The model under review builds one solid part; all positions refer to its coordinate system, in mm. Round coordinates to 2 decimals unless told otherwise and drop trailing zeros. Loops run counter-clockwise (first coordinate to the right, second up) from the corner with the lowest first, then second, coordinate; pieces in that order, holes last. Notation, with made-up numbers: M 4,-33.5 L 27,-33.5 A37 ccw 27,3.5 Z; hole C 30,32 d5. An arc over 180 degrees is marked long. Answer in a Markdown table with one row per item. Add a question column.
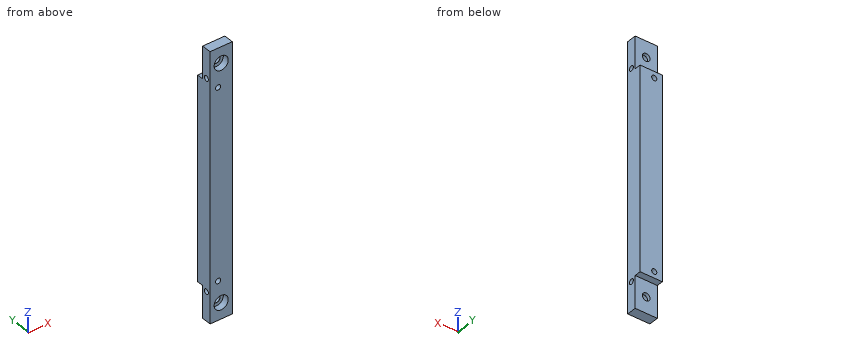
from build123d import *

# Parameters (mm, degrees)
SKETCH1_W                                      = 83
SKETCH1_H                                      = 6
BOSS_EXTRUDE1_DEPTH                            = 8.5
SKETCH7_W                                      = 8.5
SKETCH7_H                                      = 10
CUT_EXTRUDE6_DEPTH                             = 3
SKETCH18_W                                     = 10
SKETCH18_H                                     = 3
CUT_EXTRUDE8_DEPTH                             = 10
SKETCH21_W                                     = 63
SKETCH21_H                                     = 1
CUT_EXTRUDE9_DEPTH                             = 10
M2X0_4_TAPPED_HOLE3_D                          = 1.6
SKETCH27_W                                     = 1.6
SKETCH27_H                                     = 83
CUT_EXTRUDE12_DEPTH                            = 10
CBORE_FOR_M2_SOCKET_HEAD_CAP_SCREW1_AT_2_COUNT = 2
CBORE_FOR_M2_SOCKET_HEAD_CAP_SCREW1_AT_2_PITCH = 73
M2X0_4_TAPPED_HOLE2_D                          = 1.6


with BuildPart() as part:
    # Sketch1 → Boss-Extrude1 (new body)
    with BuildSketch(Plane(origin=(0, 0, 0), x_dir=(0, 0, -1), z_dir=(1, 0, 0))):
        with Locations((41.5, -5.098419508)):
            Rectangle(SKETCH1_W, SKETCH1_H)
    extrude(amount=BOSS_EXTRUDE1_DEPTH)

    # Sketch7 → Cut-Extrude6 (cut)
    with BuildSketch(Plane(origin=(0, -2.098419508, 0), x_dir=(1, 0, 0), z_dir=(0, 1, 0))):
        with Locations((4.25, 5)):
            Rectangle(SKETCH7_W, SKETCH7_H)
    extrude(amount=-CUT_EXTRUDE6_DEPTH, mode=Mode.SUBTRACT)

    # Sketch18 → Cut-Extrude8 (cut)
    with BuildSketch(Plane(origin=(8.5, 0, 0), x_dir=(0, 0, -1), z_dir=(1, 0, 0))):
        with Locations((78, -3.598419508)):
            Rectangle(SKETCH18_W, SKETCH18_H)
    extrude(amount=-CUT_EXTRUDE8_DEPTH, mode=Mode.SUBTRACT)

    # Sketch21 → Cut-Extrude9 (cut)
    with BuildSketch(Plane.ZY):
        with Locations((-41.5, -2.598419508)):
            Rectangle(SKETCH21_W, SKETCH21_H)
    extrude(amount=-CUT_EXTRUDE9_DEPTH, mode=Mode.SUBTRACT)

    # M2x0.4 Tapped Hole3 (through all)
    with Locations(Plane.ZY):
        with Locations((-74, -6.598419508), (-9, -6.598419508)):
            Hole(M2X0_4_TAPPED_HOLE3_D / 2)

    # Sketch27 → Cut-Extrude12 (cut)
    with BuildSketch(Plane.XZ.offset(8.098419508)):
        with Locations((0.8, -41.5)):
            Rectangle(SKETCH27_W, SKETCH27_H)
    extrude(amount=-CUT_EXTRUDE12_DEPTH, mode=Mode.SUBTRACT)

    # Sketch31 → CBORE for M2 Socket Head Cap Screw1 (revolve, cut)
    with BuildSketch(Plane(origin=(5.05, -8.098419508, -5), x_dir=(0, 0, -1), z_dir=(1, 0, 0))):
        Polygon((0, 0), (0, 5), (1.2, 5), (1.2, 2.025), (1.225, 2), (2.2, 2), (2.2, 0), align=None)
    cbore_for_m2_socket_head_cap_screw1 = revolve(axis=Axis((5.05, -14.448419508, -5), (0, 1, 0)), mode=Mode.SUBTRACT)

    # CBORE for M2 Socket Head Cap Screw1 at 2: CBORE for M2 Socket Head Cap Screw1 ×2
    with Locations(*[(0, 0, -i * CBORE_FOR_M2_SOCKET_HEAD_CAP_SCREW1_AT_2_PITCH) for i in range(1, CBORE_FOR_M2_SOCKET_HEAD_CAP_SCREW1_AT_2_COUNT)]):
        add(cbore_for_m2_socket_head_cap_screw1, mode=Mode.SUBTRACT)

    # M2x0.4 Tapped Hole2 (through all)
    with Locations(Plane(origin=(0, -8.098419508, 0), x_dir=(-1, 0, 0), z_dir=(0, -1, 0))):
        with Locations((-4.1, 71), (-4.1, 12)):
            Hole(M2X0_4_TAPPED_HOLE2_D / 2)


solid = part.part
1. Take a section at B-B, the plane y = -3.9. State the section outline as (x, z) points.
2. To check wall thickness, follow probe 1 along Z at (x, y) = (4.1, -5); probe 2 along Z at (x, y) = (5.05, -5.7); probe 3 along Z at (x, y) = (5.05, -6.5). State the ranges of each line that lie inside material, in increasing order.
3. Take a section at A-A, the plane z = -71. State the section outline as (x, y) points, and give its area (3 significant figures).
4. Take a section at C-C, the plane z = -5. State the section outline as (x, y) points (3 decimals).
5. For pin 1 Ø2 at (x, y) = (4, -4) entering from +Z; pin 2 Ø4 at (x, z) = (5.05, -5) entering from -Y; pin 3 Ø2 at (x, y) = (4, -4) entering from -Z, all flat-tipped, find the tip position at first contact; note any pin that passes through.
Check sheet entries:
| question | item | result |
|---|---|---|
| 1 | outline | M 1.6,-73 L 8.5,-73 L 8.5,-10 L 1.6,-10 Z; hole C 4.1,-71 d1.6; hole C 4.1,-12 d1.6 |
| 2 | probe 1 | z = -73 to -71.8, -70.2 to -12.8, -11.2 to -10 |
| 2 | probe 2 | z = -83 to -79.2, -76.8 to -6.2, -3.8 to 0 |
| 2 | probe 3 | z = -83 to -80.2, -75.8 to -74.79, -73.21 to -9.79, -8.21 to -7.2, -2.8 to 0 |
| 3 | outline | M 1.6,-8.1 L 3.3,-8.1 L 3.3,-3.1 L 1.6,-3.1 Z; M 4.9,-8.1 L 8.5,-8.1 L 8.5,-3.1 L 4.9,-3.1 Z |
| 3 | area | 26.5 mm^2 |
| 4 | outline | M 1.6,-8.098 L 2.85,-8.098 L 2.85,-6.098 L 3.825,-6.098 L 3.85,-6.073 L 3.85,-5.098 L 1.6,-5.098 Z; M 6.25,-6.073 L 6.275,-6.098 L 7.25,-6.098 L 7.25,-8.098 L 8.5,-8.098 L 8.5,-5.098 L 6.25,-5.098 Z |
| 5 | pin 1 | stops at z = -10 |
| 5 | pin 2 | stops at y = -6.1 |
| 5 | pin 3 | stops at z = -73 |
